Build history of the part. All positions in model axes, mm. A direction names the side the tool comes from. Round coordinates to 2 decimals unless told otherwise and drop trailing zeros. Write each loop counter-clockwise with the first axis right and the second up, starting at its lowest first coordinate (ties: lowest second). Pieces come first, ordered by that corner, then holes. Notation, with made-up numbers: (27.25, -13) -> (82.25, -13) arc R17 ccw to (82.25, 0) -> close; hole circle Ø5 at (15.5, 19.25). An arc over 180 degrees is marked (long way). Answer in a Markdown table with one row per item. Add a question column.
from build123d import *

# Parameters (mm, degrees)
F1_DEPTH      = 20
F3_DEPTH      = 25
F3_DEPTH_BACK = 20
F4_R          = 4.1
F5_DEPTH      = 5
F6_R          = 4.1
F7_DEPTH      = 5
F8_R          = 4.1
F9_DEPTH      = 5


with BuildPart() as f1:
    # F0 (on Top) → F1 (new body)
    with BuildSketch(Plane.XY):
        Polygon((7.0710678119, 7.0710678119), (0, 0), (0, -20), (6, -20), (6, -2.4852813742), (9.5563491861, 1.0710678119), (27.0710678119, 1.0710678119), (27.0710678119, 7.0710678119), align=None)
    extrude(amount=F1_DEPTH)

    # F2 (on face) → F3 (join, two sides)
    with BuildSketch(Plane.XY.offset(20)) as f3_sk:
        Polygon((5.6568542495, 5.6568542495), (3.5355339059, 3.5355339059), (17.6776695297, -10.6066017178), (19.7989898732, -8.4852813742), align=None)
        Polygon((17.6776695297, -10.6066017178), (3.5355339059, 3.5355339059), (1.4142135624, 1.4142135624), (15.5563491861, -12.7279220614), align=None)
    extrude(amount=F3_DEPTH)
    extrude(f3_sk.sketch, amount=-F3_DEPTH_BACK)

    # F4 (on face) → F5 (cut)
    with BuildSketch(Plane(origin=(0, 0, 0), x_dir=(0, -1, 0), z_dir=(-1, 0, 0))):
        with Locations((10, 10)):
            Circle(F4_R)
    extrude(amount=-F5_DEPTH, mode=Mode.SUBTRACT)

    # F6 (on face) → F7 (cut)
    with BuildSketch(Plane(origin=(0, 7.0710678119, 0), x_dir=(-1, 0, 0), z_dir=(0, 1, 0))):
        with Locations((-17.0710678119, 10)):
            Circle(F6_R)
    extrude(amount=-F7_DEPTH, mode=Mode.SUBTRACT)

    # F8 (on face) → F9 (cut)
    with BuildSketch(Plane(origin=(1.4142135624, 1.4142135624, 0), x_dir=(0.7071067812, -0.7071067812, 0), z_dir=(-0.7071067812, -0.7071067812, 0))):
        with Locations((10, 35)):
            Circle(F8_R)
    extrude(amount=-F9_DEPTH, mode=Mode.SUBTRACT)


solid = f1.part
(1) Saw through at D-D (x = 21.75). List the corners of the cut face in (y, z), plus the area to 3 significant figures.
(2) Saw through at C-C (y = -10). List the corners of the cut face in (x, z), plus the area to 3 significant figures.
(3) Mould opens along X. For faces 1 (the face through (9.96, -7.13, 22.18)), 2 (the face through (0, -14.3, 9.9)), 3 (the face through (16, 4, 20)) say: pulls with the +X half, pulls with the -X half, needs draft (parallel to the pull), parting line crosses it, or undercut.
(4) Which spindle directions (+Z, -Z, +X, -X, +Y, -Y) get a long thin tool onto all of the face, cutting with end or side? Do faces 4 (the face through (3, -9, 20)), 5 (the face through (13.284, 4.606, 8.43)), 6 (the face through (12, -2.1, 35.1)), 7 (the face through (6, -12, 10)), 8 (the face through (2.465, -5.904, 10.18)). Say none if no direction does.
(5) Saw through at B-B (y = 4.5). List the corners of the cut face in (x, z).
(6) Saw through at A-A (z = 10). List the corners of the cut face in (x, y).
(7) Probe line 1 along Z through (x, y) = (3.8, -10); line 2 along Y through (x, z) = (21.75, 15.5); line 3 along Y through (x, z) = (20.75, 9.5). List the from-to ranges inside material, lowest first.
(8) Drop flat-ended pins along their axis: P1, Ø13.5, axis at x = 18, z = 12.5, coming from the -Y side; P2, Ø2.5, axis at x = 16.5, z = 12, coming from the +Y side; P3, Ø5, axis at x = 20, y = 4, coming from the +Z side; P4, Ø2, axis at x = 9.5, y = -10, coming from the +Z side. Give the stop position or say it passes through.
Answer sheet:
| question | item | result |
|---|---|---|
| 1 | outline | (1.07, 0) -> (7.07, 0) -> (7.07, 20) -> (1.07, 20) -> close |
| 1 | area | 120 mm² |
| 2 | outline | (0, 0) -> (6, 0) -> (6, 20) -> (0, 20) -> (0, 14.1) -> (5, 14.1) -> (5, 5.9) -> (0, 5.9) -> close; (12.83, 0) -> (18.28, 0) -> (18.28, 45) -> (12.83, 45) -> close |
| 2 | area | 325 mm² |
| 3 | face 1 | undercut |
| 3 | face 2 | pulls with the -X half |
| 3 | face 3 | needs draft |
| 4 | face 4 | +Z, -X, -Y |
| 4 | face 5 | +Y |
| 4 | face 6 | none |
| 4 | face 7 | +Z, -Z, -Y |
| 4 | face 8 | -X |
| 5 | outline | (4.5, 0) -> (27.07, 0) -> (27.07, 20) -> (6.81, 20) -> (6.81, 45) -> (4.5, 45) -> close; hole circle Ø8.2 at (17.07, 10) |
| 6 | outline | (0, -20) -> (6, -20) -> (6, -3.17) -> (15.56, -12.73) -> (19.8, -8.49) -> (10.24, 1.07) -> (27.07, 1.07) -> (27.07, 7.07) -> (21.17, 7.07) -> (21.17, 2.07) -> (12.97, 2.07) -> (12.97, 7.07) -> (7.07, 7.07) -> (0, 0) -> (0, -5.9) -> (5, -5.9) -> (5, -14.1) -> (0, -14.1) -> close |
| 7 | line 1 | z = 0 to 5.9, 14.1 to 20 |
| 7 | line 2 | y = 1.07 to 7.07 |
| 7 | line 3 | y = 1.07 to 2.07 |
| 8 | P1 | stops at y = -12.73 |
| 8 | P2 | stops at y = 2.07 |
| 8 | P3 | stops at z = 20 |
| 8 | P4 | passes through |
